from build123d import *

# Parameters (mm, degrees)
F0_W     = 35
F0_H     = 22.5
F1_DEPTH = 2
F0_R     = 1.7
F2_DEPTH = 5
F3_R     = 4
F3_R_2   = 3.99999
F4_R     = 3
F5_DEPTH = 3


# Not quite as in the source:
# - a fillet or chamfer is up to 0.001 mm smaller than in the source, because OpenCascade refuses the exact size


with BuildPart() as f1:
    # F0 (on Top) → F1 (new body)
    with BuildSketch(Plane.XY):
        Rectangle(F0_W, F0_H)
    extrude(amount=F1_DEPTH)

    # F0 (on Top) → F2 (join)
    with BuildSketch(Plane.XY):
        Polygon((-19.25, -11.25), (-19.25, -19.25), (19.25, -19.25), (19.25, -11.25), (17.5, -11.25), (-17.5, -11.25), align=None)
        with Locations((-15.25, -15.25)):
            Circle(F0_R, mode=Mode.SUBTRACT)
        with Locations((15.25, -15.25)):
            Circle(F0_R, mode=Mode.SUBTRACT)
        Polygon((-19.25, 19.25), (-19.25, 11.25), (-17.5, 11.25), (17.5, 11.25), (19.25, 11.25), (19.25, 19.25), align=None)
        with Locations((-15.25, 15.25)):
            Circle(F0_R, mode=Mode.SUBTRACT)
        with Locations((15.25, 15.25)):
            Circle(F0_R, mode=Mode.SUBTRACT)
    extrude(amount=F2_DEPTH)

    # F3 (call 1 of 8: OpenCascade refuses the feature's edges together)
    f3_edges = [f1.edges().sort_by_distance(p)[0] for p in [
        (19.25, -19.25, 2.5),
    ]]
    fillet(f3_edges, radius=F3_R)

    # F3#2 (call 2 of 8) (radius 4 in the source; OpenCascade refuses exactly that, so slightly less here)
    f3_2_edges = [f1.edges().sort_by_distance(p)[0] for p in [
        (19.25, -11.25, 2.5),
    ]]
    fillet(f3_2_edges, radius=F3_R_2)

    # F3#3 (call 3 of 8)
    f3_3_edges = [f1.edges().sort_by_distance(p)[0] for p in [
        (-19.25, -19.25, 2.5),
    ]]
    fillet(f3_3_edges, radius=F3_R)

    # F3#4 (call 4 of 8)
    f3_4_edges = [f1.edges().sort_by_distance(p)[0] for p in [
        (-19.25, 11.25, 2.5),
    ]]
    fillet(f3_4_edges, radius=F3_R)

    # F3#5 (call 5 of 8)
    f3_5_edges = [f1.edges().sort_by_distance(p)[0] for p in [
        (19.25, 11.25, 2.5),
    ]]
    fillet(f3_5_edges, radius=F3_R)

    # F3#6 (call 6 of 8) (radius 4 in the source; OpenCascade refuses exactly that, so slightly less here)
    f3_6_edges = [f1.edges().sort_by_distance(p)[0] for p in [
        (19.25, 19.25, 2.5),
    ]]
    fillet(f3_6_edges, radius=F3_R_2)

    # F3#7 (call 7 of 8) (radius 4 in the source; OpenCascade refuses exactly that, so slightly less here)
    f3_7_edges = [f1.edges().sort_by_distance(p)[0] for p in [
        (-19.25, -11.25, 2.5),
    ]]
    fillet(f3_7_edges, radius=F3_R_2)

    # F3#8 (call 8 of 8) (radius 4 in the source; OpenCascade refuses exactly that, so slightly less here)
    f3_8_edges = [f1.edges().sort_by_distance(p)[0] for p in [
        (-19.25, 19.25, 2.5),
    ]]
    fillet(f3_8_edges, radius=F3_R_2)

    # F4 (on face) → F5 (cut)
    with BuildSketch(Plane.XY):
        with Locations((-15.25, -15.25)):
            Circle(F4_R)
        with Locations((15.25, -15.25)):
            Circle(F4_R)
        with Locations((15.25, 15.25)):
            Circle(F4_R)
        with Locations((-15.25, 15.25)):
            Circle(F4_R)
    extrude(amount=F5_DEPTH, mode=Mode.SUBTRACT)


solid = f1.part
Source: CAD feature listing. Evaluate the final solid. Frame: model axes, mm. A direction names the side the tool comes from. Give positions to 0.01 mm unless a question says otherwise; leave off trailing zeros. Write each loop counter-clockwise with the first axis right and the second up, starting at its lowest first coordinate (ties: lowest second). Pieces come first, ordered by that corner, then holes. Notation, with made-up numbers: M 44.5,-21.5 L 89.5,-21.5 A18 ccw 89.5,-16.5 Z; hole C -27,89.25 d10. An arc over 180 degrees is marked long. Return JSON: item names as keys, results as strings. Group by question number.
1) Pull-direction query (X, two-part tool) for faces 1 (the face through (18.109, 18.047, 2.535)), 2 (the face through (-15, 13, 3)), 3 (the face through (-18.109, 18.047, 2.535)); classes: pulls with the +X half, pulls with the -X half, needs draft (parallel to the pull), parting line crosses it, or undercut.
2) Cut plane C-C, the plane x = 14. Output: boundary loops of the cut face in (y, z).
3) Set-up query: faces 4 (the face through (12.869, -17.075, 1.479)), 5 (the face through (18.55, 12.99, 2.54)), 6 (the face through (-18.5, 12.92, 2.54)), 7 (the face through (0, -11.25, 3)). Return all of +Z, -Z, +X, -X, +Y, -Y with unobstructed straight access to the full face (end or side cutting, diameter ignored); none if empty.
4) Material intervals for line 1 along X through (y, z) = (-15.25, 3.6); line 2 along Y through (x, z) = (15.25, 4.55); line 3 along Y through (x, z) = (15.25, 1.35), sorted ascending. Write a range as [from, to].
5) Pin query (flat end, axial travel): P1, Ø3, axis at y = 2, z = 1.5, coming from the +X side; P2, Ø2, axis at y = 13, z = 3, coming from the -X side; P3, Ø1.8, axis at x = -15.5, y = -14, coming from the -Z side. Return the tip coordinate at first contact, or that it passes through.
6) Cut plane D-D, the plane x = -4. Output: boundary loops of the cut face in (y, z), plus the area to 3 significant figures.
7) Cut plane A-A, the plane z = 4.05. Give the number of separate pieces and of enclosed holes in the cut face, plus the area to 3 significant figures.
Recorded:
{
 "1": {"face 1": "pulls with the +X half", "face 2": "undercut", "face 3": "pulls with the -X half"},
 "2": {"outline": "M -19.25,0 L -17.98,0 L -17.98,3 L -16.4,3 L -16.4,5 L -19.25,5 Z; M -14.1,3 L -12.52,3 L -12.52,0 L 12.52,0 L 12.52,3 L 14.1,3 L 14.1,5 L 11.25,5 L 11.25,2 L -11.25,2 L -11.25,5 L -14.1,5 Z; M 16.4,3 L 17.98,3 L 17.98,0 L 19.25,0 L 19.25,5 L 16.4,5 Z"},
 "3": {"face 4": "-Z", "face 5": "+Z, +X", "face 6": "+Z, -X", "face 7": "+Z, +X, -X"},
 "4": {"line 1": "x = [-19.25, -16.95], [-13.55, 13.55], [16.95, 19.25]", "line 2": "y = [-19.25, -16.95], [-13.55, -11.25], [11.25, 13.55], [16.95, 19.25]", "line 3": "y = [-19.25, -18.25], [-12.25, 12.25], [18.25, 19.25]"},
 "5": {"P1": "stops at x = 17.5", "P2": "stops at x = -19.05", "P3": "stops at z = 3"},
 "6": {"outline": "M -19.25,0 L 19.25,0 L 19.25,5 L 11.25,5 L 11.25,2 L -11.25,2 L -11.25,5 L -19.25,5 Z", "area": "125 mm²"},
 "7": {"separate pieces": "2", "enclosed holes": "4", "area": "552 mm²"}
}
